Design review of the part shown in the three views and the two pictorial views. Dimensions are in mm from the part's minimum x, y and z. Round coordinates to 2 decimals unless told otherwise and drop trailing zeros. Loops run counter-clockwise (first coordinate to the right, second up) from the corner with the lowest first, then second, coordinate; pieces in that order, holes last.
1) Insertion check: pin 1 (4 mm diameter, centred on x = 7, z = 7, fed in from -Y). The pin has a flat end and moves straight along its axis. Give the tip position at first contact, or say it passes through.
2) Take a section at B-B (z = 12.5). State the section outline as (x, y) points.
3) Take a section at C-C (y = 1.5). State the section outline as (x, z) points, then the cut area to 3 significant figures.
4) Wall thickness on L1, parallel to X at y = 1.9, z = 4.5; L2, parallel to X at y = 3.25, z = 12.5; L3, parallel to X at y = 0.95, z = 11: over which ranges is each line inside the solid? List them lowest first.
5) Take a section at A-A (x = 31). State the section outline as (y, z) points, then the cut area to 3 significant figures.
6) Take a section at D-D (x = 8). State the section outline as (y, z) points, then the cut area to 3 significant figures.
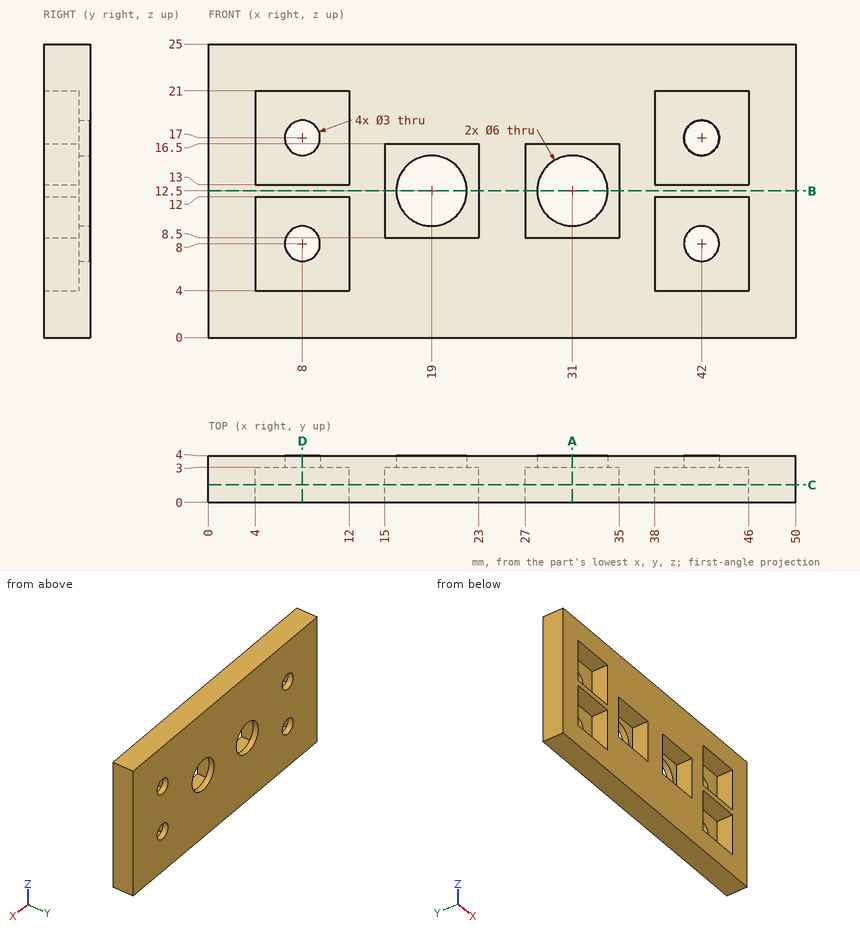
Response:
1. pin 1: stops at y = 3
2. outline: (0, 0) - (15, 0) - (15, 3) - (16, 3) - (16, 4) - (0, 4) - close; (22, 3) - (23, 3) - (23, 0) - (27, 0) - (27, 3) - (28, 3) - (28, 4) - (22, 4) - close; (34, 3) - (35, 3) - (35, 0) - (50, 0) - (50, 4) - (34, 4) - close
3. outline: (0, 0) - (50, 0) - (50, 25) - (0, 25) - close; hole (4, 4) - (12, 4) - (12, 12) - (4, 12) - close; hole (4, 13) - (12, 13) - (12, 21) - (4, 21) - close; hole (15, 8.5) - (23, 8.5) - (23, 16.5) - (15, 16.5) - close; hole (27, 8.5) - (35, 8.5) - (35, 16.5) - (27, 16.5) - close; hole (38, 4) - (46, 4) - (46, 12) - (38, 12) - close; hole (38, 13) - (46, 13) - (46, 21) - (38, 21) - close
3. area: 866 mm2
4. L1: x = 0 to 4, 12 to 38, 46 to 50
4. L2: x = 0 to 16, 22 to 28, 34 to 50
4. L3: x = 0 to 4, 12 to 15, 23 to 27, 35 to 38, 46 to 50
5. outline: (0, 0) - (4, 0) - (4, 9.5) - (3, 9.5) - (3, 8.5) - (0, 8.5) - close; (0, 16.5) - (3, 16.5) - (3, 15.5) - (4, 15.5) - (4, 25) - (0, 25) - close
5. area: 70.0 mm2
6. outline: (0, 0) - (4, 0) - (4, 6.5) - (3, 6.5) - (3, 4) - (0, 4) - close; (0, 12) - (3, 12) - (3, 9.5) - (4, 9.5) - (4, 15.5) - (3, 15.5) - (3, 13) - (0, 13) - close; (0, 21) - (3, 21) - (3, 18.5) - (4, 18.5) - (4, 25) - (0, 25) - close
6. area: 46.0 mm2
